Build history of the part. All positions in model axes, mm. A direction names the side the tool comes from. Round coordinates to 2 decimals unless told otherwise and drop trailing zeros. Loops run counter-clockwise (first coordinate to the right, second up) from the corner with the lowest first, then second, coordinate; pieces in that order, holes last. Notation, with made-up numbers: (-28, 59) - (29, 59) arc R11 ccw to (29, 76) - close; hole circle Ø9 at (76, -27.5). An arc over 180 degrees is marked (long way). Answer as CSV lines item,"result". Start each with the question number.
Autodesk Inventor part; units mm, degrees
ref_plane "YZ Plane" through (0, 0, 0) normal (1, 0, 0) x (0, 1, 0)
ref_plane "XZ Plane" through (0, 0, 0) normal (0, 1, 0) x (-1, 0, 0)
ref_plane "XY Plane" through (0, 0, 0) normal (0, 0, 1) x (1, 0, 0)
sketch "Sketch1" plane through (0, 0, 0) normal (0, 1, 0) x (-1, 0, 0)
  line L0 (-59.69, 24.765) -> (59.69, 24.765)
  line L1 (59.69, 24.765) -> (59.69, -24.765)
  line L2 (59.69, -24.765) -> (-59.69, -24.765)
  line L3 (-59.69, -24.765) -> (-59.69, 24.765)
  point P0 (0, 0)
  dimension "d0" = 119.38
  dimension "d1" = 49.53
  dimension "d2" = 24.765
  dimension "d22" = 59.69
extrude "Extrusion1" add sketch "Sketch1" along normal blind 40.64
sketch "Sketch2" plane through (0, 40.64, 0) normal (0, 1, 0) x (1, 0, 0)
  line L0 (-59.69, -24.765) -> (-39.37, -24.765)
  line L1 (-39.37, -24.765) -> (-39.37, 24.765)
  line L2 (-39.37, 24.765) -> (-59.69, 24.765)
  line L3 (-59.69, 24.765) -> (-59.69, -24.765)
  line L4 (59.69, -24.765) -> (59.69, 24.765)
  line L5 (59.69, -24.765) -> (39.37, -24.765)
  line L6 (39.37, -24.765) -> (39.37, 24.765)
  line L7 (39.37, 24.765) -> (59.69, 24.765)
  line L8 (59.69, 24.765) -> (59.69, -24.765)
  point P0 (0, 0)
  point P1 (59.69, 24.765)
  dimension "d6" = 20.32
  dimension "d7" = 20.32
  dimension "d8" = 49.53
  dimension "d9" = 49.53
  dimension "d10" = 78.74
extrude "Extrusion2" cut sketch "Sketch2" against normal blind 22.86
sketch "Sketch3" plane through (0, 0, 0) normal (0, -1, 0) x (1, 0, 0)
  circle A0 centre (50.165, 0) radius 3.175
  circle A1 centre (-50.165, 0) radius 3.175
  line L0 (-59.69, -24.765) -> (-59.69, 24.765)
  line L1 (59.69, 24.765) -> (59.69, -24.765)
  point P0 (0, 0)
  dimension "d13" = 6.35
  dimension "d14" = 6.35
  dimension "d15" = 6.35
extrude "Extrusion3" cut sketch "Sketch3" against normal blind 22.86
sketch "Sketch4" plane through (0, 0, 0) normal (0, -1, 0) x (1, 0, 0)
  line L0 (-57.15, -22.225) -> (57.15, -22.225)
  line L1 (57.15, -22.225) -> (57.15, 22.225)
  line L2 (57.15, 22.225) -> (-57.15, 22.225)
  line L3 (-57.15, 22.225) -> (-57.15, -22.225)
  line L4 (-59.69, -24.765) -> (-59.69, 24.765)
  line L5 (59.69, 24.765) -> (59.69, -24.765)
  line L6 (-59.69, 24.765) -> (59.69, 24.765)
  line L7 (59.69, -24.765) -> (-59.69, -24.765)
  point P0 (0, 0)
  dimension "d18" = 2.54
  dimension "d19" = 2.54
  dimension "d20" = 2.54
  dimension "d21" = 2.54
extrude "Extrusion4" cut sketch "Sketch4" against normal blind 15.24 contours L3 L2 L1 L0
sketch "Sketch5" plane through (0, 15.24, 0) normal (0, -1, 0) x (1, 0, 0)
  line L0 (-57.15, 22.225) -> (57.15, 22.225)
  line L1 (-36.83, -22.225) -> (36.83, -22.225)
  line L2 (36.83, -22.225) -> (36.83, 22.225)
  line L3 (36.83, 22.225) -> (-36.83, 22.225)
  line L4 (-36.83, 22.225) -> (-36.83, -22.225)
  line L5 (-36.83, -22.225) -> (36.83, 22.225) construction
  line L6 (36.83, -22.225) -> (-36.83, 22.225) construction
  point P0 (0, 0)
  dimension "d25" = 73.66
extrude "Extrusion5" cut sketch "Sketch5" against normal blind 22.86
sketch "Sketch6" plane through (0, 0, 0) normal (0, -1, 0) x (1, 0, 0)
  line L0 (58.42, -23.495) -> (-58.42, 23.495) construction
  line L1 (-58.42, -23.495) -> (58.42, 23.495) construction
  line L2 (-59.69, -24.765) -> (-59.69, 24.765)
  line L3 (-59.69, 24.765) -> (59.69, 24.765)
  line L4 (50.165, 23.495) -> (50.165, 24.765)
  line L5 (-50.165, 23.495) -> (-50.165, 24.765)
  line L6 (-58.42, 15.24) -> (-59.69, 15.24)
  line L7 (-58.42, -15.24) -> (-59.69, -15.24)
  line L8 (-50.165, -23.495) -> (-50.165, -24.765)
  line L9 (50.165, -23.495) -> (50.165, -24.765)
  line L10 (59.69, -24.765) -> (-59.69, -24.765)
  line L11 (59.69, 24.765) -> (59.69, -24.765)
  line L12 (59.69, -15.24) -> (58.42, -15.24)
  line L13 (59.69, 15.24) -> (58.42, 15.24)
  line L14 (-50.165, 24.765) -> (50.165, 24.765)
  line L15 (59.69, -15.24) -> (59.69, 15.24)
  line L16 (50.165, -24.765) -> (-50.165, -24.765)
  line L17 (-59.69, -15.24) -> (-59.69, 15.24)
  line L18 (-57.15, -22.225) -> (-57.15, 22.225)
  line L19 (57.15, 22.225) -> (-57.15, 22.225)
  line L20 (-57.15, 22.225) -> (-57.15, -22.225)
  line L21 (-57.15, -22.225) -> (57.15, -22.225)
  line L22 (57.15, -22.225) -> (57.15, 22.225)
  line L23 (57.15, 22.225) -> (-57.15, -22.225) construction
  line L24 (-57.15, 22.225) -> (57.15, -22.225) construction
  line L25 (-58.42, -23.495) -> (-58.42, -15.24)
  line L26 (-58.42, 15.24) -> (-58.42, 23.495)
  line L27 (-58.42, 23.495) -> (-50.165, 23.495)
  line L28 (50.165, 23.495) -> (58.42, 23.495)
  line L29 (58.42, 23.495) -> (58.42, 15.24)
  line L30 (58.42, -15.24) -> (58.42, -23.495)
  line L31 (58.42, -23.495) -> (50.165, -23.495)
  line L32 (-50.165, -23.495) -> (-58.42, -23.495)
  point P0 (0, 0)
  point P1 (-59.055, 15.24)
  point P2 (-59.055, -15.24)
  dimension "d30" = 100.33
  dimension "d31" = 50.165
  dimension "d32" = 30.48
  dimension "d33" = 15.24
  dimension "d34" = 30.48
  dimension "d35" = 15.24
  dimension "d40" = 100.33
  dimension "d41" = 50.165
extrude "Extrusion6" cut sketch "Sketch6" against normal blind 2.54 contours L2 L6 L26 L27 L5 L3 L4 L28 L29 L13 L11 L12 L30 L31 L9 L10 L8 L32 L25 L7 | L18 L19 L22 L21
sketch "Sketch7" plane through (0, 2.54, 0) normal (0, -1, 0) x (1, 0, 0)
  line L0 (-36.83, 22.225) -> (36.83, 22.225)
  line L1 (-39.37, 24.765) -> (39.37, 24.765)
  line L2 (34.925, 22.225) -> (-34.925, 22.225)
  line L3 (-34.925, 22.225) -> (-34.925, 24.765)
  line L4 (-34.925, 24.765) -> (34.925, 24.765)
  line L5 (34.925, 24.765) -> (34.925, 22.225)
  line L6 (50.165, -24.765) -> (-50.165, -24.765)
  line L7 (-57.15, -22.225) -> (57.15, -22.225)
  line L8 (-34.925, -24.765) -> (34.925, -24.765)
  line L9 (34.925, -24.765) -> (34.925, -22.225)
  line L10 (34.925, -22.225) -> (-34.925, -22.225)
  line L11 (-34.925, -22.225) -> (-34.925, -24.765)
  point P0 (0, 0)
  dimension "d42" = 69.85
  dimension "d43" = 34.925
  dimension "d44" = 69.85
  dimension "d45" = 34.925
extrude "Extrusion7" cut sketch "Sketch7" against normal blind 7.62
sketch "Sketch8" plane through (0, 2.54, 0) normal (0, -1, 0) x (1, 0, 0)
  line L0 (-57.15, 22.225) -> (-57.15, -22.225)
  line L1 (-59.69, -15.24) -> (-59.69, 15.24)
  line L2 (-57.15, -6.985) -> (-59.69, -6.985)
  line L3 (-59.69, -6.985) -> (-59.69, 6.985)
  line L4 (-59.69, 6.985) -> (-57.15, 6.985)
  line L5 (-57.15, 6.985) -> (-57.15, -6.985)
  point P0 (0, 0)
  dimension "d48" = 13.97
  dimension "d49" = 6.985
extrude "Extrusion8" cut sketch "Sketch8" against normal blind 10.16
mirror "Mirror1" about plane through (0, 0, 0) normal (1, 0, 0) of "Extrusion8"
fillet "Fillet1" radius 2.54 12 edges at (57.15, 8.89, 22.225) (58.42, 1.27, 23.495) (-58.42, 1.27, 23.495) (-57.15, 8.89, 22.225) (-58.42, 1.27, -23.495) (-57.15, 8.89, -22.225) (57.15, 8.89, -22.225) (58.42, 1.27, -23.495) (-59.69, 8.89, 24.765) (59.69, 8.89, 24.765) (-59.69, 8.89, -24.765) (59.69, 8.89, -24.765)
fillet "Fillet2" radius 1.27 18 edges at (-58.9461, 17.78, 24.0211) (-59.69, 17.78, 0) (-58.9461, 17.78, -24.0211) (-48.26, 17.78, -24.765) (-48.26, 17.78, 24.765) (58.9461, 17.78, 24.0211) (59.69, 17.78, 0) (58.9461, 17.78, -24.0211) (48.26, 17.78, -24.765) (48.26, 17.78, 24.765) (39.37, 29.21, 24.765) (0, 40.64, 24.765) (39.37, 40.64, 0) (39.37, 29.21, -24.765) (0, 40.64, -24.765) (-39.37, 40.64, 0) (-39.37, 29.21, 24.765) (-39.37, 29.21, -24.765)
chamfer "Chamfer1" distance 5.08 distance2 7.62 1 edges at (-34.925, 2.54, 23.495) measured on face at (-40.005, 2.54, 23.495)
chamfer "Chamfer2" distance 5.08 distance2 7.62 1 edges at (34.925, 2.54, 23.495) measured on face at (40.005, 2.54, 23.495)
chamfer "Chamfer3" distance 5.08 distance2 7.62 1 edges at (34.925, 2.54, -23.495) measured on face at (40.005, 2.54, -23.495)
chamfer "Chamfer4" distance 5.08 distance2 7.62 1 edges at (-34.925, 2.54, -23.495) measured on face at (-40.005, 2.54, -23.495)
properties part number "CO-1-01-12VoltFuseBox"
Q1. Band-saw the part on B-B, the plane y = 34. List the corners of the cut face in (x, z) (3 decimals), then the cut area to 3 significant figures.
Q2. Two-plate mould, pull along Z, no slides. Class faces 1 (the cylindrical face through (58.966, 8.371, -24.001)), 2 (the cylindrical face through (57.656, 1.288, 22.771)), 3 (the cylindrical face through (-58.966, 8.371, 24.001)): released by +Z, released by -Z, zero draft, split by the parting line, or undercut.
Q3. Wall check: probe 1 along Z at (x, y) = (-30, 14.5) (3 decimals); probe 2 along X at (y, z) = (21.5, -17); probe 3 along X at (y, z) = (11.5, -17.5). Give the ranges that are in metal, low to high. Write a range as [from, to].
Q4. Band-saw the part on D-D, the plane x = -7.5. List the corners of the cut face in (y, z) (3 decimals), then the cut area to 3 significant figures.
Q5. Band-saw the part on C-C, the plane z = 13. List the corners of the cut face in (x, y).
Q6. Pin check, flat tips, straight feed: pin 1 Ø9 at (x, z) = (45, 16.5) entering from -Y; pin 2 Ø1.5 at (y, z) = (27, -7) entering from -X; pin 3 Ø11.5 at (y, z) = (26.5, -8.5) entering from +X; pin 4 Ø3 at (x, y) = (-10.5, 8.5) entering from -Z. Stop position of each tip, or through.
Q7. Band-saw the part on A-A, the plane z = 0. List the corners of the cut face in (x, y), then the cut area to 3 significant figures.
Q8. Tool access for faces 4 (the flat face through (58, 8, -6.985)), 5 (the flat face through (-1, 38.1, 0)), 6 (the flat face through (46.6, 17.78, -0.3)): list every direction of +Z, -Z, +X, -X, +Y, -Y with a clear straight run to the whole face (end or side of a thin tool).
Reported:
1,outline,"(-39.37, -23.495) arc R1.27 ccw to (-38.1, -24.765) - (38.1, -24.765) arc R1.27 ccw to (39.37, -23.495) - (39.37, 23.495) arc R1.27 ccw to (38.1, 24.765) - (-38.1, 24.765) arc R1.27 ccw to (-39.37, 23.495) - close; hole (-36.83, -22.225) - (36.83, -22.225) - (36.83, 22.225) - (-36.83, 22.225) - close"
1,area,"624 mm2"
2,face 1,"released by -Z"
2,face 2,"undercut"
2,face 3,"released by +Z"
3,probe 1,"z = [-24.765, -22.225], [22.225, 24.765]"
3,probe 2,"x = [-39.37, -36.83], [36.83, 39.37]"
3,probe 3,"x = [-59.69, -57.15], [57.15, 59.69]"
4,outline,"(10.16, -24.765) - (39.37, -24.765) arc R1.27 ccw to (40.64, -23.495) - (40.64, 23.495) arc R1.27 ccw to (39.37, 24.765) - (10.16, 24.765) - (10.16, 22.225) - (38.1, 22.225) - (38.1, -22.225) - (10.16, -22.225) - close"
4,area,"267 mm2"
5,outline,"(-59.69, 2.54) - (-57.15, 2.54) - (-57.15, 15.24) - (-36.83, 15.24) - (-36.83, 38.1) - (36.83, 38.1) - (36.83, 15.24) - (57.15, 15.24) - (57.15, 2.54) - (59.69, 2.54) - (59.69, 16.51) arc R1.27 ccw to (58.42, 17.78) - (39.37, 17.78) - (39.37, 39.37) arc R1.27 ccw to (38.1, 40.64) - (-38.1, 40.64) arc R1.27 ccw to (-39.37, 39.37) - (-39.37, 17.78) - (-58.42, 17.78) arc R1.27 ccw to (-59.69, 16.51) - close"
6,pin 1,"stops at y = 15.24"
6,pin 2,"stops at x = -39.37"
6,pin 3,"stops at x = 39.37"
6,pin 4,"passes through"
7,outline,"(-59.69, 12.7) - (-57.15, 12.7) - (-57.15, 15.24) - (-53.34, 15.24) - (-53.34, 17.78) - (-58.42, 17.78) arc R1.27 ccw to (-59.69, 16.51) - close; (-46.99, 15.24) - (-36.83, 15.24) - (-36.83, 38.1) - (36.83, 38.1) - (36.83, 15.24) - (46.99, 15.24) - (46.99, 17.78) - (39.37, 17.78) - (39.37, 39.37) arc R1.27 ccw to (38.1, 40.64) - (-38.1, 40.64) arc R1.27 ccw to (-39.37, 39.37) - (-39.37, 17.78) - (-46.99, 17.78) - close; (53.34, 15.24) - (57.15, 15.24) - (57.15, 12.7) - (59.69, 12.7) - (59.69, 16.51) arc R1.27 ccw to (58.42, 17.78) - (53.34, 17.78) - close"
7,area,"399 mm2"
8,face 4,"+X, -X, -Y"
8,face 5,"-Y"
8,face 6,"+Z, -Z, +X, +Y"
